CAD build for the part. Positions are in the model's coordinates, mm. A direction names the side the tool comes from. Coordinates: 2 decimals unless noted, no trailing zeros. Loops run counter-clockwise (first coordinate to the right, second up) from the corner with the lowest first, then second, coordinate; pieces in that order, holes last. Notation, with made-up numbers: (-6.5, 73.5) -> (22.5, 73.5) arc R14 cw to (22.5, 78.5) -> close; hole circle Ø7 at (-15, 38). An arc over 180 degrees is marked (long way). Return JSON: item names as keys, results as strings. Group by question number.
(1) Flat gauge pins, fed straight in: pin 1 Ø1.5 at (y, z) = (10.5, -5.5) entering from +X; pin 2 Ø3 at (x, z) = (35, -1.5) entering from +Y; pin 3 Ø1.5 at (x, z) = (24, -7.5) entering from +Y. Where does each tip first touch, or does it go through?
(2) Mould opens along Z. For faces 3 (the face through (-47.53, 0.82, 2.46)), 4 (the face through (-6.47, 49.58, -3.55)), 5 (the face through (-4, 46, -7)), 6 (the face through (-1, 46, 5)) say: pulls with the +Z half, pulls with the -Z half, needs draft (parallel to the pull), parting line crosses it, or undercut.
(3) Probe L1, parallel to Z at x = -46, y = 10.5; L2, parallel to X at y = 14.5, z = -5.5; L3, parallel to X at y = 15, z = -1.75. List the from-to ranges inside material, lowest first.
(4) Saw through at A-A on y = 24. Write the cut outline in (x, z).
(5) Saw through at D-D on x = -41.5. Write the cut outline in (y, z), then the cut area to 3 significant figures.
(6) Tool access for faces 1 (the face through (-47.53, 0.82, -9.54)), 2 (the face through (-4, 46, 0)): list every direction of +Z, -Z, +X, -X, +Y, -Y with a clear straight run to the whole face (end or side of a thin tool).
(7) Saw through at C-C on y = 49. Write the cut outline in (x, z).
(8) Saw through at B-B on z = 1.5. Write the cut outline in (x, y), then the cut area to 3 significant figures.
```python
from build123d import *

# Parameters (mm, degrees)
SKETCH1_W                    = 50
SKETCH1_H                    = 7
REVOLVE1_ANGLE               = 167.5
SHELL7_T                     = 5
CUT_EXTRUDE1_DEPTH           = 80.617837197
CUT_EXTRUDE1_DEPTH_BACK      = 10
CUT_EXTRUDE2_DEPTH           = 80.617837197
CUT_EXTRUDE2_DEPTH_BACK      = 10
CUT_EXTRUDE3_DEPTH           = 80.617837197
CUT_EXTRUDE3_DEPTH_BACK      = 10
CUT_EXTRUDE4_DEPTH           = 80.617837197
CUT_EXTRUDE4_DEPTH_BACK      = 10
CUT_EXTRUDE_THIN2_DEPTH      = 80.617837197
CUT_EXTRUDE_THIN2_DEPTH_BACK = 20
CUT_EXTRUDE_THIN3_DEPTH      = 80.617837197
CUT_EXTRUDE_THIN3_DEPTH_BACK = 20


with BuildPart() as part:
    # Sketch1 → Revolve1 (revolve)
    with BuildSketch(Plane(origin=(0, 0, 0), x_dir=(1, 0, 0), z_dir=(0, 1, 0))):
        with Locations((-25, 3.5)):
            Rectangle(SKETCH1_W, SKETCH1_H)
    revolve(axis=Axis((0, 0, 0), (0, 0, -1)), revolution_arc=REVOLVE1_ANGLE)

    # Shell7
    shell7_openings = [part.faces().sort_by_distance(p)[0] for p in [
        (-25, 0, -3.5),
        (24.407400178, 5.410990348, -3.5),
    ]]
    offset(amount=SHELL7_T, openings=shell7_openings, kind=Kind.INTERSECTION)

    # Sketch2 → Cut-Extrude1 (cut, two sides: drawn at the far end of the back side and taken through both)
    with BuildSketch(Plane.XY.offset(5).offset(-CUT_EXTRUDE1_DEPTH_BACK)):
        Polygon((-307.130564413, -27.612787673), (-55, 0), (53.696280392, 11.904178767), (305.826844804, 39.51696644), (361.05242015, -464.744162386), (-251.904989067, -531.873916498), align=None)
    extrude(amount=CUT_EXTRUDE1_DEPTH + CUT_EXTRUDE1_DEPTH_BACK, mode=Mode.SUBTRACT)

    # Sketch4 → Cut-Extrude2 (cut, two sides: drawn at the far end of the back side and taken through both)
    with BuildSketch(Plane(origin=(0, 0, -12), x_dir=(-1, 0, 0), z_dir=(0, 0, -1)).offset(-CUT_EXTRUDE2_DEPTH_BACK)):
        Polygon((-305.826844804, 39.51696644), (-53.696280392, 11.904178767), (55, 0), (307.130564413, -27.612787673), (251.904989067, -531.873916498), (-361.05242015, -464.744162386), align=None)
    extrude(amount=CUT_EXTRUDE2_DEPTH + CUT_EXTRUDE2_DEPTH_BACK, mode=Mode.SUBTRACT)

    # Sketch5 → Cut-Extrude3 (cut, two sides: drawn at the far end of the back side and taken through both)
    with BuildSketch(Plane.XY.offset(5).offset(-CUT_EXTRUDE3_DEPTH_BACK)):
        with BuildLine():
            Line((-50.710864423, -233.723704503), (-44.986635536, 1.096641764))
            ThreePointArc((-44.986635536, 1.096641764), (-4.899009368, 44.73253522), (43.682915928, 10.807537003))
            Line((43.682915928, 10.807537003), (100.095882825, -217.207679557))
            Line((100.095882825, -217.207679557), (151.239386336, -684.19567653))
            Line((151.239386336, -684.19567653), (0.432639088, -700.711701476))
            Line((0.432639088, -700.711701476), (-50.710864423, -233.723704503))
        make_face()
    extrude(amount=CUT_EXTRUDE3_DEPTH + CUT_EXTRUDE3_DEPTH_BACK, mode=Mode.SUBTRACT)

    # Sketch6 → Cut-Extrude4 (cut, two sides: drawn at the far end of the back side and taken through both)
    with BuildSketch(Plane(origin=(0, 0, -12), x_dir=(-1, 0, 0), z_dir=(0, 0, -1)).offset(-CUT_EXTRUDE4_DEPTH_BACK)):
        with BuildLine():
            Line((-100.095882825, -217.207679557), (-43.682915928, 10.807537003))
            ThreePointArc((-43.682915928, 10.807537003), (4.899009368, 44.73253522), (44.986635536, 1.096641764))
            Line((44.986635536, 1.096641764), (50.710864423, -233.723704503))
            Line((50.710864423, -233.723704503), (-0.432639088, -700.711701476))
            Line((-0.432639088, -700.711701476), (-151.239386336, -684.19567653))
            Line((-151.239386336, -684.19567653), (-100.095882825, -217.207679557))
        make_face()
    extrude(amount=CUT_EXTRUDE4_DEPTH + CUT_EXTRUDE4_DEPTH_BACK, mode=Mode.SUBTRACT)

    # Sketch13 → Cut-Extrude-Thin2 (cut, two sides: drawn at the far end of the back side and taken through both)
    with BuildSketch(Plane.XY.offset(5).offset(-CUT_EXTRUDE_THIN2_DEPTH_BACK)):
        Polygon((48.68959816, 11.355857885), (46.775458357, 28.833743654), (56.716021739, 29.922412403), (58.630161542, 12.444526633), align=None)
    extrude(amount=CUT_EXTRUDE_THIN2_DEPTH + CUT_EXTRUDE_THIN2_DEPTH_BACK, mode=Mode.SUBTRACT)

    # Sketch14 → Cut-Extrude-Thin3 (cut, two sides: drawn at the far end of the back side and taken through both)
    with BuildSketch(Plane.XY.offset(5).offset(-CUT_EXTRUDE_THIN3_DEPTH_BACK)):
        Polygon((-49.99699777, 0.547917856), (-51.927891207, 17.96441574), (-61.8669959, 16.862509251), (-59.936102463, -0.553988632), align=None)
    extrude(amount=CUT_EXTRUDE_THIN3_DEPTH + CUT_EXTRUDE_THIN3_DEPTH_BACK, mode=Mode.SUBTRACT)


solid = part.part
```
Geometry results:
{
 "1": {"pin 1": "x = -48.72", "pin 2": "y = 43.62", "pin 3": "y = 49.84"},
 "2": {"face 3": "needs draft", "face 4": "undercut", "face 5": "undercut", "face 6": "pulls with the +Z half"},
 "3": {"L1": "-12 to -7, 0 to 5", "L2": "-51.54 to -47.85, 47.85 to 48.35", "L3": "-51.6 to -47.7, 47.7 to 48.29"},
 "4": {"outline": "(-49.49, -12) -> (-38.07, -12) -> (-38.07, -7) -> (-43.86, -7) -> (-43.86, 0) -> (-38.07, 0) -> (-38.07, 5) -> (-49.49, 5) -> close; (38.07, -12) -> (47.3, -12) -> (47.3, 5) -> (38.07, 5) -> (38.07, 0) -> (43.86, 0) -> (43.86, -7) -> (38.07, -7) -> close"},
 "5": {"outline": "(17.4, -12) -> (36.09, -12) -> (36.09, 5) -> (17.4, 5) -> (17.4, 0) -> (27.89, 0) -> (27.89, -7) -> (17.4, -7) -> close", "area": "244 mm²"},
 "6": {"face 1": "+Z, -Z, +X, -Y", "face 2": "-Y"},
 "7": {"outline": "(-24.98, -12) -> (24.98, -12) -> (24.98, 5) -> (-24.98, 5) -> close; hole (-9.95, -7) -> (9.95, -7) -> (9.95, 0) -> (-9.95, 0) -> close"},
 "8": {"outline": "(-51.99, 17.96) -> (-51.93, 17.96) -> (-50, 0.55) -> (-44.99, 1.1) arc R45 cw to (43.68, 10.81) -> (48.69, 11.36) -> (46.78, 28.83) -> (46.83, 28.84) arc R55 ccw to start", "area": "1,340 mm²"}
}
